from build123d import *

# Parameters (mm, degrees)
SKETCH1_W           = 44.958
SKETCH1_H           = 304.8
BOSS_EXTRUDE1_DEPTH = 8.89
SKETCH2_W           = 8.89
SKETCH2_H           = 101.6
BOSS_EXTRUDE2_DEPTH = 6.35
SKETCH3_W           = 222.25
SKETCH3_H           = 6.35
BOSS_EXTRUDE3_DEPTH = 38.608


with BuildPart() as part:
    # Sketch1 → Boss-Extrude1 (new body)
    with BuildSketch(Plane.XY):
        with Locations((-6.477, 3.048)):
            Rectangle(SKETCH1_W, SKETCH1_H)
        with BuildLine():
            Line((-3.302, 133.858), (-3.302, -143.002))
            Line((-3.302, -143.002), (3.302, -143.002))
            Line((3.302, -143.002), (3.302, 143.002))
            Line((3.302, 143.002), (-16.256, 143.002))
            Line((-16.256, 143.002), (-16.256, 136.398))
            Line((-16.256, 136.398), (-5.842, 136.398))
            ThreePointArc((-5.842, 136.398), (-4.045948776, 135.654051224), (-3.302, 133.858))
        make_face(mode=Mode.SUBTRACT)
    extrude(amount=BOSS_EXTRUDE1_DEPTH)

    # Sketch2 → Boss-Extrude2 (add)
    with BuildSketch(Plane(origin=(16.002, 0, 0), x_dir=(0, 0, -1), z_dir=(1, 0, 0))):
        Polygon((222.25, -60.452), (222.25, -47.752), (0, -47.752), (0, -149.352), (222.25, -149.352), (222.25, -136.652), (228.6, -136.652), (228.6, -119.718666667), (222.25, -119.718666667), (222.25, -107.018666667), (228.6, -107.018666667), (228.6, -90.085333333), (222.25, -90.085333333), (222.25, -77.385333333), (228.6, -77.385333333), (228.6, -60.452), align=None)
        with BuildLine():
            ThreePointArc((11.4, -116.592), (9.9, -118.092), (8.4, -116.592))
            Line((8.4, -116.592), (8.4, -111.512))
            ThreePointArc((8.4, -111.512), (9.9, -110.012), (11.4, -111.512))
            Line((11.4, -111.512), (11.4, -116.592))
        make_face(mode=Mode.SUBTRACT)
        with BuildLine():
            Line((42.4, -111.512), (42.4, -116.592))
            ThreePointArc((42.4, -116.592), (40.9, -118.092), (39.4, -116.592))
            Line((39.4, -116.592), (39.4, -111.512))
            ThreePointArc((39.4, -111.512), (40.9, -110.012), (42.4, -111.512))
        make_face(mode=Mode.SUBTRACT)
        with BuildLine():
            ThreePointArc((36.4, -101.092), (25.4, -112.092), (14.4, -101.092))
            Line((14.4, -101.092), (14.4, -96.012))
            ThreePointArc((14.4, -96.012), (25.4, -85.012), (36.4, -96.012))
            Line((36.4, -96.012), (36.4, -101.092))
        make_face(mode=Mode.SUBTRACT)
        with BuildLine():
            ThreePointArc((11.4, -85.592), (9.9, -87.092), (8.4, -85.592))
            Line((8.4, -85.592), (8.4, -80.512))
            ThreePointArc((8.4, -80.512), (9.9, -79.012), (11.4, -80.512))
            Line((11.4, -80.512), (11.4, -85.592))
        make_face(mode=Mode.SUBTRACT)
        with BuildLine():
            ThreePointArc((42.4, -85.592), (40.9, -87.092), (39.4, -85.592))
            Line((39.4, -85.592), (39.4, -80.512))
            ThreePointArc((39.4, -80.512), (40.9, -79.012), (42.4, -80.512))
            Line((42.4, -80.512), (42.4, -85.592))
        make_face(mode=Mode.SUBTRACT)
        with Locations((-4.445, -98.552)):
            Rectangle(SKETCH2_W, SKETCH2_H)
    extrude(amount=-BOSS_EXTRUDE2_DEPTH)

    # Sketch3 → Boss-Extrude3 (add)
    with BuildSketch(Plane.ZY.offset(-9.652)):
        with Locations((-111.125, -146.177)):
            Rectangle(SKETCH3_W, SKETCH3_H)
    extrude(amount=BOSS_EXTRUDE3_DEPTH)


solid = part.part
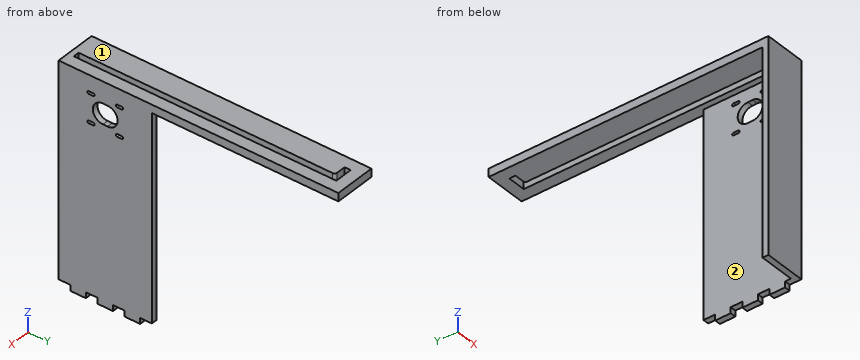
Part model, mm, in its own coordinate system. Face numbers are marked on the shaded views. A direction names the side the tool comes from. Give positions to 0.01 mm unless a question says otherwise; leave off trailing zeros. Loops run counter-clockwise (first coordinate to the right, second up) from the corner with the lowest first, then second, coordinate; pieces in that order, holes last.
(1) 3-axis set-ups, long thin cutter, end or side, ignore diameter. For the marked faces 1 and 2: which of +Z, -Z, +X, -X, +Y, -Y reach the whole face in a straight line?
Return value:
face 1: +Z, +X, -X, +Y, -Y
face 2: -Z, -X, +Y
(2) Band-saw the part on B-B (x = -13). Write the cut outline in (y, z).
Return value:
outline: (-149.35, -222.25) - (-143, -222.25) - (-143, 0) - (136.4, 0) - (136.4, 8.89) - (-149.35, 8.89) - close; (143, 0) - (155.45, 0) - (155.45, 8.89) - (143, 8.89) - close
(3) Band-saw the part on A-A (y = -36). Write the cut outline in (x, z).
Return value:
outline: (-28.96, 0) - (-3.3, 0) - (-3.3, 8.89) - (-28.96, 8.89) - close; (3.3, 0) - (16, 0) - (16, 8.89) - (3.3, 8.89) - close
(4) Band-saw the part on C-C (z = -25.4). Write the cut outline in (x, y), and give its area (3 significant figures).
Return value:
outline: (-28.96, -149.35) - (16, -149.35) - (16, -112.09) - (9.65, -112.09) - (9.65, -143) - (-28.96, -143) - close; (9.65, -85.01) - (16, -85.01) - (16, -47.75) - (9.65, -47.75) - close
area: 718 mm2
(5) Pin check, flat tips, straight feed: pin 1 (14 mm diameter, centred on x = 1.5, y = -143.5, fed in from -Z); pin 2 (7 mm diameter, centred on x = 14, z = -226, fed in from -Y); pin 3 (10 mm diameter, centred on x = -14, y = -18, fed in from -Z). Stop position of each tip, or through.
Return value:
pin 1: stops at z = -222.25
pin 2: stops at y = -136.65
pin 3: stops at z = 0
(6) Drill centre lines: line 1 along Y through (x, z) = (-13, -124); line 2 along Z through (x, y) = (6, -84); line 3 along X through (y, z) = (-65, -176). Where is each one in solid material? Low to high.
Return value:
line 1: y = -149.35 to -143
line 2: z = 0 to 8.89
line 3: x = 9.65 to 16
(7) Band-saw the part on D-D (z = -72.5). Write the cut outline in (x, y), and give its area (3 significant figures).
Return value:
outline: (-28.96, -149.35) - (16, -149.35) - (16, -47.75) - (9.65, -47.75) - (9.65, -143) - (-28.96, -143) - close
area: 890 mm2
